```python
from build123d import *

# Parameters (mm, degrees)
BOX019_W          = 28.5
BOX019_H          = 10
BOX019_DEPTH      = 20
BOX020_W          = 22
BOX020_H          = 10
BOX020_DEPTH      = 33
BOX021_W          = 28.5
BOX021_H          = 10
BOX021_DEPTH      = 23
BOX024_W          = 26.2
BOX024_H          = 60
BOX024_DEPTH      = 2.2
BOX025_W          = 22
BOX025_H          = 60
BOX025_DEPTH      = 17
CYLINDER008_R     = 1.8
CYLINDER008_DEPTH = 30
CYLINDER009_R     = 1.8
CYLINDER009_DEPTH = 30
BOX026_W          = 29
BOX026_H          = 13
BOX026_DEPTH      = 15
BOX027_W          = 22
BOX027_H          = 25
BOX027_DEPTH      = 15
BOX022_W          = 12.6
BOX022_H          = 20
BOX022_DEPTH      = 12
BOX018_W          = 22
BOX018_H          = 10
BOX018_DEPTH      = 29
BOX014_W          = 80
BOX014_H          = 1.5
BOX014_DEPTH      = 79.5
BOX023_W          = 32
BOX023_H          = 64
BOX023_DEPTH      = 20
BOX015_W          = 74
BOX015_H          = 2
BOX015_DEPTH      = 77


with BuildPart() as pc:
    # Box019 → Box019 (new body)
    with BuildSketch(Plane(origin=(43, 0, 54), x_dir=(1, 0, 0), z_dir=(0, 0, 1))):
        with Locations((14.25, 5)):
            Rectangle(BOX019_W, BOX019_H)
    extrude(amount=BOX019_DEPTH)


with BuildPart() as obj1:
    # Box020 → Box020 (new body)
    with BuildSketch(Plane(origin=(47, -7.5, 10), x_dir=(1, 0, 0), z_dir=(0, 0, 1))):
        with Locations((11, 5)):
            Rectangle(BOX020_W, BOX020_H)
    extrude(amount=BOX020_DEPTH)


with BuildPart() as pc001:
    # Box021 → Box021 (new body)
    with BuildSketch(Plane(origin=(43, -7.3, 52.5), x_dir=(1, 0, 0), z_dir=(0, 0, 1))):
        with Locations((14.25, 5)):
            Rectangle(BOX021_W, BOX021_H)
    extrude(amount=BOX021_DEPTH)


with BuildPart() as obj2:
    # Box024 → Box024 (new body)
    with BuildSketch(Plane(origin=(35.9, -3.5, 51), x_dir=(-1, 0, 0), z_dir=(0, 0, 1))):
        with Locations((13.1, 30)):
            Rectangle(BOX024_W, BOX024_H)
    extrude(amount=BOX024_DEPTH)


with BuildPart() as obj3:
    # Box025 → Box025 (new body)
    with BuildSketch(Plane(origin=(34, -3.5, 49), x_dir=(-1, 0, 0), z_dir=(0, 0, 1))):
        with Locations((11, 30)):
            Rectangle(BOX025_W, BOX025_H)
    extrude(amount=BOX025_DEPTH)


with BuildPart() as cylinder008:
    # Cylinder008 → Cylinder008 (new body)
    with BuildSketch(Plane(origin=(34, -58, 38), x_dir=(1, 0, 0), z_dir=(0, 0, 1))):
        Circle(CYLINDER008_R)
    extrude(amount=CYLINDER008_DEPTH)


with BuildPart() as cylinder009:
    # Cylinder009 → Cylinder009 (new body)
    with BuildSketch(Plane(origin=(12, -58, 38), x_dir=(1, 0, 0), z_dir=(0, 0, 1))):
        Circle(CYLINDER009_R)
    extrude(amount=CYLINDER009_DEPTH)


with BuildPart() as obj4:
    # Box026 → Box026 (new body)
    with BuildSketch(Plane(origin=(8.5, -65.5, 53.2), x_dir=(1, 0, 0), z_dir=(0, 0, 1))):
        with Locations((14.5, 6.5)):
            Rectangle(BOX026_W, BOX026_H)
    extrude(amount=BOX026_DEPTH)


with BuildPart() as obj5:
    # Box027 → Box027 (new body)
    with BuildSketch(Plane(origin=(12, -53.5, 65.2), x_dir=(1, 0, 0), z_dir=(0, 0, 1))):
        with Locations((11, 12.5)):
            Rectangle(BOX027_W, BOX027_H)
    extrude(amount=BOX027_DEPTH)


with BuildPart() as obj6:
    # Box022 → Box022 (new body)
    with BuildSketch(Plane(origin=(16.7, -9, 53), x_dir=(1, 0, 0), z_dir=(0, 0, 1))):
        with Locations((6.3, 10)):
            Rectangle(BOX022_W, BOX022_H)
    extrude(amount=BOX022_DEPTH)

    # Fusion006: union obj2, obj3, Cylinder008, Cylinder009, obj4, obj5
    add(obj2.part)
    add(obj3.part)
    add(cylinder008.part)
    add(cylinder009.part)
    add(obj4.part)
    add(obj5.part)


with BuildPart() as fusion004:
    # Box018 → Box018 (new body)
    with BuildSketch(Plane(origin=(47, -6.5, 12), x_dir=(1, 0, 0), z_dir=(0, 0, 1))):
        with Locations((11, 5)):
            Rectangle(BOX018_W, BOX018_H)
    extrude(amount=BOX018_DEPTH)

    # Fusion004: union PC, obj1, PC001, obj6
    add(pc.part)
    add(obj1.part)
    add(pc001.part)
    add(obj6.part)


with BuildPart() as cube014:
    # Box014 → Box014 (new body)
    with BuildSketch(Plane(origin=(0, 2, 0.5), x_dir=(1, 0, 0), z_dir=(0, 0, 1))):
        with Locations((40, 0.75)):
            Rectangle(BOX014_W, BOX014_H)
    extrude(amount=BOX014_DEPTH)


with BuildPart() as obj7:
    # Box023 → Box023 (new body)
    with BuildSketch(Plane(origin=(39, 1, 47), x_dir=(-1, 0, 0), z_dir=(0, 0, 1))):
        with Locations((16, 32)):
            Rectangle(BOX023_W, BOX023_H)
    extrude(amount=BOX023_DEPTH)


with BuildPart() as obj8:
    # Box015 → Box015 (new body)
    with BuildSketch(Plane(origin=(3, 1, 3), x_dir=(1, 0, 0), z_dir=(0, 0, 1))):
        with Locations((37, 1)):
            Rectangle(BOX015_W, BOX015_H)
    extrude(amount=BOX015_DEPTH)

    # Fusion005: union Cube014, obj7
    add(cube014.part)
    add(obj7.part)

    # Cut002: cut Fusion004
    add(fusion004.part, mode=Mode.SUBTRACT)


solid = obj8.part
```
Here's how the part is built. I have some questions about the finished solid (model axes, mm). A direction names the side the tool comes from. Give positions to 0.01 mm unless a question says otherwise; leave off trailing zeros. Loops run counter-clockwise (first coordinate to the right, second up) from the corner with the lowest first, then second, coordinate; pieces in that order, holes last. Notation, with made-up numbers: M 27.25,18.25 L 72.25,18.25 A17 ccw 72.25,50.25 Z; hole C 44.5,56.5 d4. An arc over 180 degrees is marked long. Return JSON: item names as keys, results as strings.
Item 1: Imagine slicing it at D-D on x = 52.5. List the corners of the cut face in (y, z) for me, then the cut area to 4 significant figures.
A:
{"outline": "M 1,3 L 2,3 L 2,0.5 L 3.5,0.5 L 3.5,12 L 2.5,12 L 2.5,10 L 1,10 Z; M 1,43 L 2.5,43 L 2.5,41 L 3.5,41 L 3.5,54 L 2.7,54 L 2.7,52.5 L 1,52.5 Z; M 1,75.5 L 2.7,75.5 L 2.7,74 L 3.5,74 L 3.5,80 L 1,80 Z", "area": "62.65 mm^2"}
Item 2: I'm going to push flat-ended pins straight in: pin 1 Ø8 at (x, z) = (42.5, 44) entering from -Y; pin 2 Ø6 at (y, z) = (-18.5, 57.5) entering from -X; pin 3 Ø16 at (y, z) = (-43, 61) entering from +X; pin 4 Ø3 at (y, z) = (2.5, 30.5) entering from -X. Where does each tip first touch, or does it pass through?
A:
{"pin 1": "stops at y = 1", "pin 2": "stops at x = 7", "pin 3": "stops at x = 39", "pin 4": "stops at x = 0"}
Item 3: Imagine slicing it at A-A on z = 59. List the corners of the cut face in (x, y) for me.
A:
{"outline": "M 0,2 L 3,2 L 3,1 L 7,1 L 7,-63 L 8.5,-63 L 8.5,-52.5 L 12,-52.5 L 12,-3.5 L 16.7,-3.5 L 16.7,3.5 L 0,3.5 Z; M 29.3,-3.5 L 34,-3.5 L 34,-52.5 L 37.5,-52.5 L 37.5,-63 L 39,-63 L 39,1 L 43,1 L 43,3.5 L 29.3,3.5 Z; M 71.5,1 L 77,1 L 77,2 L 80,2 L 80,3.5 L 71.5,3.5 Z"}
Item 4: Please list where these lines run through material, in increasing order: line 1 (X direction, y = -58, z = 48.4); line 2 (Y direction, x = 12, z = 48.55); line 3 (X direction, y = -58, z = 50).
A:
{"line 1": "x = 7 to 10.2, 13.8 to 32.2, 35.8 to 39", "line 2": "y = -63 to -59.8, -56.2 to 3.5", "line 3": "x = 7 to 10.2, 35.8 to 39"}
Item 5: On a 3-axis mill with a long thin cutter (end or side, diameter ignored), from which of +Z, -Z, +X, -X, +Y, -Y can I reach the whole of each face in a straight line? I mean faces 5 (the flat face through (34, -28, 60)), 6 (the flat face through (23, 0, 65)), 7 (the flat face through (34, -61, 50)). Say none if no direction works.
A:
{"face 5": "-Y", "face 6": "+Y, -Y", "face 7": "+Z, -Y"}
Item 6: Imagine slicing it at B-B on z = 38. List the corners of the cut face in (x, y) for me.
A:
{"outline": "M 0,2 L 3,2 L 3,1 L 47,1 L 47,3.5 L 0,3.5 Z; M 69,1 L 77,1 L 77,2 L 80,2 L 80,3.5 L 69,3.5 Z"}
Item 7: Thinking about a two-plate mould opening in X: for faces 1 (the flat face through (7, -31, 57)), 2 (the flat face through (11, -28, 53.2)), 3 (the flat face through (43, 2, 64)), 4 (the flat face through (23, -17, 67)), which applies, released by +X, released by -X, zero draft, split by the parting line, or undercut?
A:
{"face 1": "released by -X", "face 2": "undercut", "face 3": "undercut", "face 4": "zero draft"}
Item 8: Imagine slicing it at C-C on y = -58. List the corners of the cut face in (x, z) for me.
A:
{"outline": "M 7,47 L 10.2,47 L 10.2,51 L 9.7,51 L 9.7,53.2 L 8.5,53.2 L 8.5,67 L 7,67 Z; M 13.8,47 L 32.2,47 L 32.2,49 L 13.8,49 Z; M 35.8,47 L 39,47 L 39,67 L 37.5,67 L 37.5,53.2 L 35.9,53.2 L 35.9,51 L 35.8,51 Z"}
